Design review of the part shown in the three views and the two pictorial views. Dimensions are in mm from the part's minimum x, y and z. A direction names the side the tool comes from. Coordinates: 2 decimals unless noted, no trailing zeros. Order: outer loops, then holes, each group sorted by start corner. A loop starts at its lowest first (then second) coordinate and runs counter-clockwise, first axis right, second up. Notation, with made-up numbers: (8, 29.25) -> (24, 29.25) arc R9 ccw to (24, 44.25) -> close; hole circle Ø8 at (19, 37.5). An arc over 180 degrees is marked (long way). Answer as a JSON object with one key per item and string values. Group by question number.
1) For pin 1 (4 mm diameter, centred on x = 5.5, z = 6, fed in from -Y); pin 2 (1.5 mm diameter, centred on x = 11, z = 14, fed in from -Y) (1 decimal); pin 3 (2 mm diameter, centred on x = 11.5, z = 11, fed in from -Y); pin 4 (8 mm diameter, centred on y = 8.5, z = 12, fed in from -X), all flat-tipped, find the tip position at first contact; note any pin that passes through.
2) Wall thickness on L1, parallel to X at y = 2.5, z = 11 (1 decimal); L2, parallel to Y at x = 8.5, z = 11 (1 decimal); L3, parallel to X at y = 12.25, z = 15 (1 decimal): over which ranges is each line inside the solid? List them lowest first.
3) Machinability: for the marked faces 1, 2 and 3, which of the approach directions +Z, -Z, +X, -X, +Y, -Y give a long, thin tool a straight path to every point of the face, cutting with its end or side? Answer none if there is none.
4) Draft analysis for pull direction Y (two halves, no side actions). For the marked faces 4, 5, 6 and 7, state which applies: +Y half, -Y half, draft (parallel to the pull), parting line (faces both ways), or undercut.
5) Add section D-D, the plane y = 13.5. Write out the cut boundary in (x, z) (1 decimal).
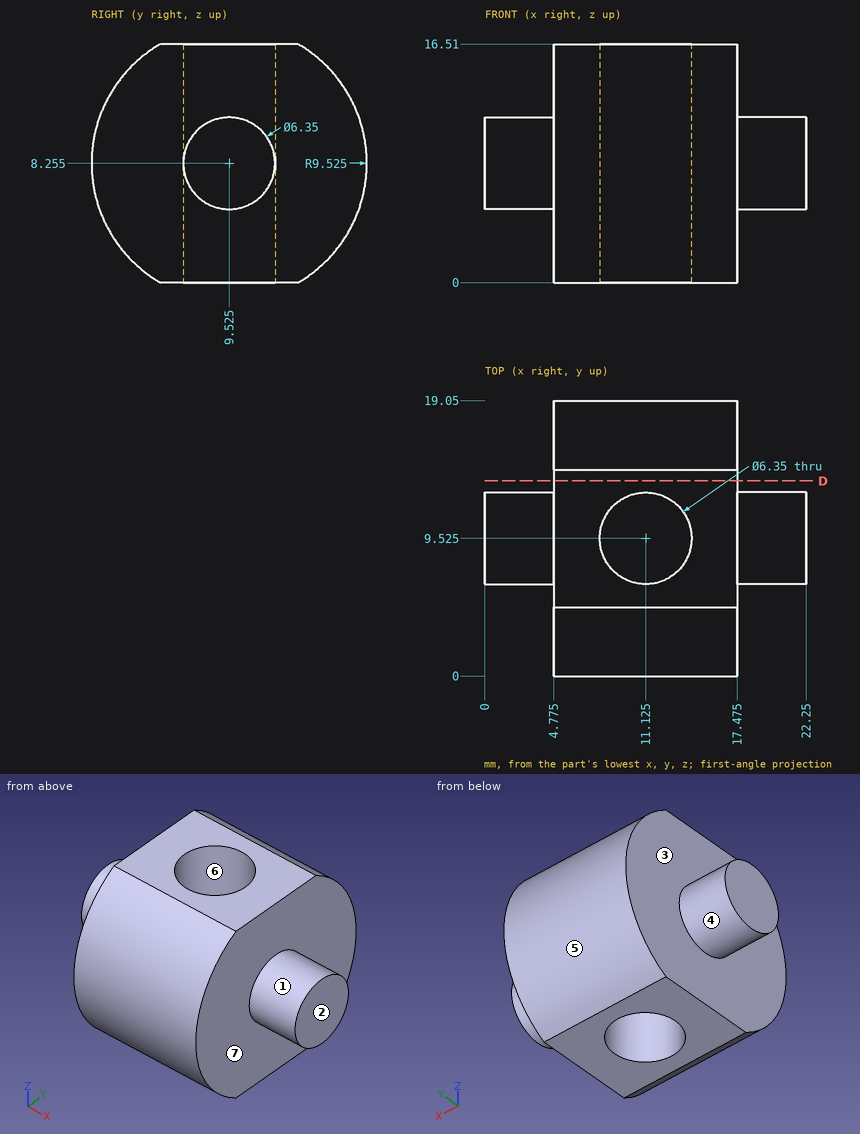
Output values:
{
 "1": {"pin 1": "stops at y = 0", "pin 2": "stops at y = 1.4", "pin 3": "stops at y = 0.16", "pin 4": "stops at x = 0"},
 "2": {"L1": "x = 4.8 to 17.5", "L2": "y = 0.4 to 7.7, 11.3 to 18.6", "L3": "x = 4.8 to 9.5, 12.8 to 17.5"},
 "3": {"face 1": "+X", "face 2": "+Z, -Z, +X, +Y, -Y", "face 3": "-X"},
 "4": {"face 4": "parting line", "face 5": "+Y half", "face 6": "undercut", "face 7": "draft"},
 "5": {"outline": "(4.8, 0) -> (17.5, 0) -> (17.5, 16.5) -> (4.8, 16.5) -> close"}
}
